Autodesk Inventor part; units mm, degrees
ref_plane "Work Plane1" through (-84, 2, -178) normal (-1, 0, 0) x (0, 0, 1)
ref_plane "YZ Plane" through (0, 0, 0) normal (1, 0, 0) x (0, 1, 0)
ref_plane "XZ Plane" through (0, 0, 0) normal (0, 1, 0) x (-1, 0, 0)
sketch "Sketch1" plane through (0, 0, 0) normal (0, 1, 0) x (-1, 0, 0)
  line L0 (0, 0) -> (180, 0)
  line L1 (180, 0) -> (180, -180)
  line L2 (180, -180) -> (0, -180)
  line L3 (0, -180) -> (0, 0)
  dimension "d0" = 180
  dimension "d1" = 180
extrude "Extrusion1" add sketch "Sketch1" along normal blind 2
sketch "Sketch4" plane through (0, 2, 0) normal (0, 1, 0) x (1, 0, 0)
  line L0 (0, 180) -> (-180, 180)
  line L1 (-180, 180) -> (-180, 0)
  line L2 (0, 180) -> (-180, 180)
  line L3 (-180, 180) -> (-180, 178)
  line L4 (-180, 178) -> (0, 178)
  line L5 (0, 178) -> (0, 180)
  line L6 (-180, 0) -> (0, 0)
  line L7 (0, 0) -> (-180, 0)
  line L8 (-180, 0) -> (-180, 2)
  line L9 (-180, 2) -> (0, 2)
  line L10 (0, 2) -> (0, 0)
  line L11 (0, 2) -> (-2, 2)
  line L12 (-2, 2) -> (-2, 178)
  line L13 (-2, 178) -> (0, 178)
  line L14 (0, 178) -> (0, 2)
  line L15 (-180, 178) -> (-178, 178)
  line L16 (-178, 178) -> (-178, 2)
  line L17 (-178, 2) -> (-180, 2)
  line L18 (-180, 2) -> (-180, 178)
  dimension "d16" = 2
  dimension "d17" = 2
  dimension "d18" = 2
  dimension "d19" = 2
extrude "Extrusion4" add sketch "Sketch4" along normal blind 36 contours L5 L4 L1 L0 | L14 L9 L12 L4 | L4 L16 L9 L1 | L10 L6 L1 L9
sketch "Sketch5" plane through (0, 2, 0) normal (0, 1, 0) x (1, 0, 0)
  circle A0 centre (-174, 6) radius 1.65
  circle A1 centre (-174, 174) radius 1.65
  circle A2 centre (-6, 174) radius 1.65
  circle A3 centre (-6, 6) radius 1.65
  point P0 (0, 0)
  dimension "d22" = 3.3
  dimension "d23" = 3.3
  dimension "d24" = 3.3
  dimension "d25" = 3.3
extrude "Extrusion5" cut sketch "Sketch5" against normal through all
sketch "Sketch8" plane through (-180, 0, -180) normal (-1, 0, 0) x (0, 0, 1)
  line L0 (178, 2) -> (2, 2)
  line L1 (143.5, 14) -> (107.5, 14)
  line L2 (107.5, 14) -> (107.5, 2)
  line L3 (107.5, 2) -> (143.5, 2)
  line L4 (143.5, 2) -> (143.5, 14)
  line L5 (178, 2) -> (178, 38)
  point P0 (180, 0)
  point P1 (143.5, 2)
  point P2 (107.5, 2)
  dimension "d84" = 36
  dimension "d101" = 12
  dimension "d108" = 34.5
extrude "Extrusion10" cut sketch "Sketch8" against normal blind 10
sketch "Sketch15" plane through (-2, 2, -2) normal (-1, 0, 0) x (0, 0, 1)
  line L0 (-141.5, 17.33) -> (-133.04, 17.33) construction
  line L1 (-112.2541, 3.188) -> (-128.2862, 2.9082)
  arc A0 (-141.5, 8.8698) -> (-128.2862, 2.9082) centre (-129.027, 18.891) ccw
  arc A1 (-112.2541, 3.188) -> (-88, 17.33) centre (-104.25, 17.33) ccw
  line L2 (-112.2541, 31.472) -> (-128.2862, 31.7518)
  arc A2 (-128.2862, 31.7518) -> (-141.5, 25.7902) centre (-129.027, 15.769) ccw
  arc A3 (-88, 17.33) -> (-112.2541, 31.472) centre (-104.25, 17.33) ccw
  line L3 (-141.5, 17.33) -> (-141.5, 8.8698)
  line L4 (-141.5, 17.33) -> (-141.5, 25.7902)
  line L5 (-176, 36) -> (0, 36)
  line L6 (0, 0) -> (-176, 0)
  point P0 (2, -2)
extrude "Extrusion17" cut sketch "Sketch15" against normal through all
ref_plane "Work Plane1" through (-84, 2, -178) normal (-1, 0, 0) x (0, 0, 1)
sketch "Sketch16" plane through (-84, 2, -178) normal (-1, 0, 0) x (0, 0, 1)
  arc A0 (63.7459, 3.188) -> (63.7459, 31.472) centre (71.75, 17.33) ccw
  line L0 (176, 0) -> (0, 0)
  line L1 (71.75, 0) -> (79.5, 0)
  line L2 (-2, -2) -> (178, -2)
  line L3 (45.25, 0) -> (53, 0) construction
  line L4 (79.5, 0) -> (79.5, 6.2762)
  line L5 (71.75, 0) -> (64, 0)
  line L6 (45.25, 0) -> (53, 0) construction
  line L7 (64, 0) -> (64, 6.2762)
  arc A1 (61.4422, 22.429) -> (82.0578, 22.429) centre (71.75, 17.33) ccw
  line L8 (59.25, 22.429) -> (61.4422, 22.429)
  line L9 (82.0578, 22.429) -> (84.25, 22.429)
  arc A2 (59.25, 22.429) -> (64, 6.2762) centre (71.75, 17.33) ccw
  arc A3 (79.5, 6.2762) -> (84.25, 22.429) centre (71.75, 17.33) ccw
  dimension "d135" = 23
extrude "Extrusion18" add sketch "Sketch16" along normal blind 4
sketch "Sketch17" plane through (0, 0, 0) normal (1, 0, 0) x (0, 0, -1)
  line L0 (36.5, 2) -> (2, 2)
  line L1 (53, 2) -> (88, 2)
  line L2 (88, 2) -> (88, 23.37)
  line L3 (88, 23.37) -> (53, 23.37)
  line L4 (53, 23.37) -> (53, 2)
  line L5 (0, 0) -> (0, 38)
  arc A0 (61.49, 20.185) -> (61.49, 4.185) centre (61.49, 12.185) ccw
  arc A1 (77.4348, 3.2471) -> (77.4348, 21.1229) centre (78.49, 12.185) ccw
  line L6 (78.49, 3.185) -> (61.49, 4.185)
  line L7 (78.49, 21.185) -> (61.49, 20.185)
  dimension "d144" = 35
  dimension "d145" = 21.37
  dimension "d147" = 16
  dimension "d148" = 18
extrude "Extrusion19" cut sketch "Sketch17" against normal blind 10 contours L7 A1 L6 A0
sketch "Sketch21" plane through (0, 2, 0) normal (0, 1, 0) x (1, 0, 0)
  circle A0 centre (-17.39, 69.81) radius 1.05
  circle A1 centre (-33.79, 69.81) radius 1.05
  point P0 (0, 0)
  dimension "d155" = 2.1
  dimension "d156" = 2.1
extrude "Extrusion21" add sketch "Sketch21" along normal blind 6
sketch "Sketch22" plane through (0, 2, 0) normal (0, 1, 0) x (1, 0, 0)
  line L0 (-36, 88) -> (-31, 88)
  line L1 (-31, 88) -> (-31, 90)
  line L2 (-31, 90) -> (-36, 90)
  line L3 (-36, 90) -> (-36, 88)
  line L4 (-31, 53) -> (-36, 53)
  line L5 (-36, 53) -> (-36, 51)
  line L6 (-36, 51) -> (-31, 51)
  line L7 (-31, 51) -> (-31, 53)
  line L8 (-2, 2) -> (-2, 178)
  line L9 (-2, 90) -> (-178, 90) construction
  line L10 (-178, 178) -> (-178, 72.5)
  point P0 (0, 0)
  dimension "d159" = 5
  dimension "d160" = 2
  dimension "d161" = 5
  dimension "d162" = 2
extrude "Extrusion22" add sketch "Sketch22" along normal blind 23
sketch "Sketch23" plane through (-36, 2, -88) normal (0, 0, 1) x (1, 0, 0)
  line L0 (5, 0) -> (5, 23)
  line L1 (5, 23) -> (0, 23)
  line L2 (0, 23) -> (0, 21)
  line L3 (0, 21) -> (5, 21)
  line L4 (5, 21) -> (5, 23)
  point P0 (36, -2)
  dimension "d165" = 5
  dimension "d166" = 2
sketch "Sketch24" plane through (-31, 2, -53) normal (0, 0, -1) x (-1, 0, 0)
  line L0 (0, 23) -> (5, 23)
  line L1 (5, 23) -> (5, 21)
  line L2 (5, 21) -> (0, 21)
  line L3 (0, 21) -> (0, 23)
  point P0 (-31, -2)
  dimension "d167" = 5
  dimension "d168" = 2
extrude "Extrusion23" add sketch "Sketch23" along normal blind 2.4
extrude "Extrusion24" add sketch "Sketch24" along normal blind 2.4
sketch "Sketch25" plane through (-36, 23, -88) normal (0, -1, 0) x (1, 0, 0)
  line L0 (5, 0) -> (0, 0)
  line L1 (0, 0) -> (0, 1.2)
  line L2 (0, 1.2) -> (5, 1.2)
  line L3 (5, 1.2) -> (5, 0)
  point P0 (36, 88)
  dimension "d173" = 5
  dimension "d174" = 1.2
sketch "Sketch26" plane through (-36, 23, -53) normal (0, -1, 0) x (1, 0, 0)
  line L0 (5, 0) -> (0, 0)
  line L1 (0, 0) -> (0, -1.2)
  line L2 (0, -1.2) -> (5, -1.2)
  line L3 (5, -1.2) -> (5, 0)
  point P0 (36, 53)
  dimension "d175" = 5
  dimension "d176" = 1.2
extrude "Extrusion25" cut sketch "Sketch26" against normal blind 1
extrude "Extrusion26" cut sketch "Sketch25" against normal blind 1
fillet "Fillet1" radius 2.5 2 edges at (-33.5, 23, -85.6) (-33.5, 23, -55.4)
properties part number "base plate"
Input: part model. Units: mm. Frame: model coordinates. A direction names the side the tool comes from. Give positions to 0.01 mm unless a question says otherwise; leave off trailing zeros. Order: outer loops, then holes, each group sorted by start corner. A loop starts at its lowest first (then second) coordinate and runs counter-clockwise, first axis right, second up. Notation, with made-up numbers: (-9.75, 82.25) -> (47.25, 82.25) arc R17 ccw to (47.25, 112.25) -> close; hole circle Ø3 at (59, 69). An arc over 180 degrees is marked (long way). Use one line per item in the form item = value.
1) Section A-A, the plane z = -146. Return loops of the section in (x, y).
Response values:
outline = (-180, 0) -> (0, 0) -> (0, 38) -> (-2, 38) -> (-2, 2) -> (-178, 2) -> (-178, 38) -> (-180, 38) -> close
2) Line query: probe 1 along Z at (x, y) = (-174, 0.7); probe 2 along Z at (x, y) = (-107, 35.5). Output: solid intervals per line, ascending.
Response values:
probe_1 = -180 to -175.65, -172.35 to -7.65, -4.35 to 0
probe_2 = -180 to -178, -2 to 0
3) Section C-C, the plane x = -78. Return loops of the section in (y, z).
Response values:
outline = (0, -180) -> (38, -180) -> (38, -178) -> (2, -178) -> (2, -2) -> (38, -2) -> (38, 0) -> (0, 0) -> close
4) First-contact query: pin 1 Ø0.7 at (x, z) = (-85.5, -95) entering from +Y; pin 2 Ø3.5 at (y, z) = (11.5, -53.5) entering from -X; pin 3 Ø2 at (y, z) = (5, -80.5) entering from +X. Flat tips, straight axial feed; report the tip coordinate or a pass-through.
Response values:
pin_1 = 24.43
pin_2 = -36
pin_3 = -178
5) Section B-B, the plane z = -83. Return loops of the section in (x, y), and give its area (3 significant figures).
Response values:
outline = (-180, 0) -> (0, 0) -> (0, 4.4) -> (-2, 4.4) -> (-2, 2) -> (-178, 2) -> (-178, 38) -> (-180, 38) -> close; (-2, 19.97) -> (0, 19.97) -> (0, 38) -> (-2, 38) -> close
area = 473 mm^2
6) Reachability of faces 1 (the flat face through (-36, 14, -52)), 2 (the flat face through (-33, 13, -53)), 3 (the cylindrical face through (-1.01, 6.35, -137.7)), 4 (the flat face through (-91, 19, -180)) from +Z, -Z, +X, -X, +Y, -Y: full face, straight path, thin tool, end or side. Return the list, or none.
Response values:
face_1 = +Y
face_2 = none
face_3 = +X
face_4 = -Z, +X, -X, +Y, -Y
7) Mould query, pull axis X, two halves, no side actions, for faces 5 (the flat face through (0, 27, -91)), 6 (the cylindrical face through (-1.014, 33.247, -97.861)), 7 (the flat face through (-33, 25, -53)). Classes: pulls with the +X half, pulls with the -X half, needs draft (parallel to the pull), parting line crosses it, or undercut.
Response values:
face_5 = pulls with the +X half
face_6 = needs draft
face_7 = undercut
